The listing builds one solid part. Answer for the finished solid, in the listing's coordinates (mm). A direction names the side the tool comes from. Coordinates: 2 decimals unless noted, no trailing zeros. Loops run counter-clockwise (first coordinate to the right, second up) from the corner with the lowest first, then second, coordinate; pieces in that order, holes last. Notation, with made-up numbers: (88.5, 43.5) - (116.5, 43.5) arc R30 ccw to (116.5, 81.5) - close; hole circle Ø7 at (-38.75, 40). An arc over 180 degrees is marked (long way). One line per question, with ' | ' between items.
from build123d import *

# Parameters (mm, degrees)
F0_W     = 90
F0_H     = 50
F1_DEPTH = 54
F2_W     = 20
F2_H     = 44
F3_DEPTH = 50.001
F4_SIZE  = 22
F6_DEPTH = 50.001
F7_R     = 5
F8_DEPTH = 25


with BuildPart() as f1:
    # F0 (on Top) → F1 (new body)
    with BuildSketch(Plane.XY):
        Rectangle(F0_W, F0_H)
    extrude(amount=F1_DEPTH)

    # F2 (on face) → F3 (cut, through all)
    with BuildSketch(Plane.XZ.offset(25)):
        with Locations((-35, 32)):
            Rectangle(F2_W, F2_H)
        Polygon((45, 54), (-25, 54), (45, 35.243557), align=None)
    extrude(amount=-F3_DEPTH, mode=Mode.SUBTRACT)

    # F4
    f4_edges = [f1.edges().sort_by_distance(p)[0] for p in [
        (10, -25, 44.621778),
        (10, 25, 44.621778),
    ]]
    chamfer(f4_edges, length=F4_SIZE)

    # F5 (on face) → F6 (cut, through all)
    with BuildSketch(Plane.XZ.offset(25)):
        Polygon((61.415475, 42.577509), (18, 42.577509), (61.007772, 17.74696), align=None)
    extrude(amount=-F6_DEPTH, mode=Mode.SUBTRACT)

    # F7 (on face) → F8 (cut)
    with BuildSketch(Plane.XY.offset(10)):
        with Locations((-35, 12.5)):
            Circle(F7_R)
        with Locations((-35, -12.5)):
            Circle(F7_R)
    extrude(amount=-F8_DEPTH, mode=Mode.SUBTRACT)


solid = f1.part
Item 1: Find section B-B, the plane y = -2. Write down the section's boundary in (x, z).
Taken from the geometry:
outline: (-45, 0) - (45, 0) - (45, 26.99) - (18.32, 42.39) - (-25, 54) - (-25, 10) - (-45, 10) - close
Item 2: Which of the six approach directions +Z, -Z, +X, -X, +Y, -Y give full straight-line access (tool end or side, diameter ignored) to faces 4 (the face through (-39.995, 12.72, 5.07)), 5 (the face through (-25, 0, 27))?
Taken from the geometry:
face 4: +Z, -Z | face 5: +Z, -X, +Y, -Y
Item 3: Find the intervals of material crossed by line 1 (Y direction, x = -35, z = 3.25); line 2 (X direction, y = 5.5, z = 20.5); line 3 (Z direction, x = -32.5, y = 17), in increasing order. Write a range as [from, to].
Taken from the geometry:
line 1: y = [-25, -17.5], [-7.5, 7.5], [17.5, 25] | line 2: x = [-25, 45] | line 3: z = [0, 10]
Item 4: The mould has two halves that part along X. Classify faces 1 (the face through (-1, 25, 12)), 2 (the face through (-39.995, -12.28, 5.07)), 3 (the face through (-45, 0, 5)): pulls with the +X half, pulls with the -X half, needs draft (parallel to the pull), parting line crosses it, or undercut.
Taken from the geometry:
face 1: needs draft | face 2: undercut | face 3: pulls with the -X half
Item 5: Find section A-A, the plane x = -35. Write down the section's boundary in (y, z), plus the area to 3 significant figures.
Taken from the geometry:
outline: (-25, 0) - (-17.5, 0) - (-17.5, 10) - (-25, 10) - close; (-7.5, 0) - (7.5, 0) - (7.5, 10) - (-7.5, 10) - close; (17.5, 0) - (25, 0) - (25, 10) - (17.5, 10) - close | area: 300 mm2
Item 6: Find section C-C, the plane y = -13.5. Write down the section's boundary in (x, z), plus the area to 3 significant figures.
Taken from the geometry:
outline: (-45, 0) - (-39.9, 0) - (-39.9, 10) - (-45, 10) - close; (-30.1, 0) - (45, 0) - (45, 24.37) - (-25, 43.13) - (-25, 10) - (-30.1, 10) - close | area: 2,460 mm2
Item 7: Each of these flat-tipped pins is pushed along its axis until it touches: pin 1 Ø4 at (x, y) = (0, -9) entering from +Z; pin 2 Ø10 at (y, z) = (6, 44.5) entering from +X; pin 3 Ø11.5 at (x, y) = (-35, -12.5) entering from +Z; pin 4 Ø2 at (x, y) = (30, -11) entering from -Z. Where does it stop, or does it pass through?
Taken from the geometry:
pin 1: stops at z = 43.23 | pin 2: stops at x = 22.85 | pin 3: stops at z = 10 | pin 4: stops at z = 0
Item 8: Find section D-D, the plane x = 24. Write down the section's boundary in (y, z), plus the area to 3 significant figures.
Taken from the geometry:
outline: (-25, 0) - (25, 0) - (25, 18.09) - (4.7, 39.11) - (-4.7, 39.11) - (-25, 18.09) - close | area: 1,530 mm2
